from build123d import *

# Parameters (mm, degrees)
SKETCH1_R           = 213.710950615
BOSS_EXTRUDE1_DEPTH = 12
CUT_EXTRUDE1_START  = -6.405003169
CUT_EXTRUDE1_DEPTH  = 6.405003169
CIRPATTERN1_COUNT   = 5


with BuildPart() as part:
    # Sketch1 → Boss-Extrude1 (new body)
    with BuildSketch(Plane.XY):
        Circle(SKETCH1_R)
    extrude(amount=BOSS_EXTRUDE1_DEPTH)

    # Sketch2 → Cut-Extrude1 (cut)
    with BuildSketch(Plane.XY.offset(12).offset(CUT_EXTRUDE1_START)):
        with BuildLine():
            Line((-47.040542179, 100.736288781), (47.040542179, 100.736288781))
            Line((47.040542179, 100.736288781), (107.884686522, 184.48106902))
            ThreePointArc((107.884686522, 184.48106902), (0, 213.710950615), (-107.884686522, 184.48106902))
            Line((-107.884686522, 184.48106902), (-47.040542179, 100.736288781))
        make_face()
    cut_extrude1 = extrude(amount=CUT_EXTRUDE1_DEPTH, mode=Mode.SUBTRACT)

    # CirPattern1: Cut-Extrude1 ×5 about axis
    cirpattern1_axis = Axis((0, 0, 0), (0, 0, 1))
    for i in range(1, CIRPATTERN1_COUNT):
        add(cut_extrude1.rotate(cirpattern1_axis, i * 360 / CIRPATTERN1_COUNT), mode=Mode.SUBTRACT)


solid = part.part
CAD build for the part. Positions are in the model's coordinates, mm. A direction names the side the tool comes from. Round coordinates to 2 decimals unless told otherwise and drop trailing zeros. Loops run counter-clockwise (first coordinate to the right, second up) from the corner with the lowest first, then second, coordinate; pieces in that order, holes last.
(1) Cut at B-B (x = 0). Give the cut face in (y, z) (3 decimals), plus the area to 3 significant figures.
(2) Which spindle directions (+Z, -Z, +X, -X, +Y, -Y) get a long thin tool onto all of the face, cutting with end or side? Do faces 1 (the flat face through (77.037, 142.022, 8.753)), 2 (the flat face through (-151, 47, 5.595)), 3 (the flat face through (158.88, -29.38, 8.75)), 4 (the flat face through (-92, -129, 5.595)). Say none if no direction does.
(3) Cut at A-A (z = 8.5). Give the cut face in (x, y).
(4) Cut at C-C (y = -40.5). Give the cut face in (x, z) (3 decimals), plus the area to 3 significant figures.
(5) Two-plate mould, pull along X, no slides. Class faces 5 (the flat face through (-3, 3, 0)), 6 (the flat face through (-96.01, 30.5, 8.75)), 7 (the flat face through (-2, 158, 5.595)): +X half, -X half, draft (parallel to the pull), parting line (faces both ways), or undercut.
(6) Wall check: line 1 along Z through (x, y) = (-85, -68.5) (3 decimals); line 2 along X through (y, z) = (-168, 8); line 3 along Y through (x, z) = (-1, 11.25). Give the ranges that are in metal, low to high.
(7) Cut at D-D (x = 153.5). Give the cut face in (y, z) (3 decimals).
(8) Drop flat-ended pins along their axis: pin 1 (1.9 mm diameter, centred on y = -140, z = 8, fed in from +X); pin 2 (1 mm diameter, centred on x = -120.5, y = 53, fed in from +Z) (3 decimals); pin 3 (7 mm diameter, centred on y = -175, z = 8.5, fed in from -X); pin 4 (1.5 mm diameter, centred on x = 35, y = 155, fed in from -Z). Give the stop position or say it passes through.
Findings below:
1. outline: (-213.711, 0) - (213.711, 0) - (213.711, 5.595) - (100.736, 5.595) - (100.736, 12) - (-213.711, 12) - close
1. area: 4,410 mm2
2. face 1: +Z, +Y
2. face 2: +Z, -X
2. face 3: +Z, +X
2. face 4: +Z, -Y
3. outline: (-208.79, -45.6) arc R213.71 ccw to (-195.72, -85.84) - (-97.27, -53.85) - (-21.15, -109.15) - (-21.15, -212.66) arc R213.71 ccw to (21.15, -212.66) - (21.15, -109.15) - (97.27, -53.85) - (195.72, -85.84) arc R213.71 ccw to (208.79, -45.6) - (110.34, -13.61) - (81.27, 75.87) - (142.11, 159.61) arc R213.71 ccw to (107.88, 184.48) - (47.04, 100.74) - (-47.04, 100.74) - (-107.88, 184.48) arc R213.71 ccw to (-142.11, 159.61) - (-81.27, 75.87) - (-110.34, -13.61) - close
4. outline: (-209.838, 0) - (209.838, 0) - (209.838, 5.595) - (193.104, 5.595) - (193.104, 12) - (-193.104, 12) - (-193.104, 5.595) - (-209.838, 5.595) - close
4. area: 4,820 mm2
5. face 5: draft
5. face 6: -X half
5. face 7: undercut
6. line 1: z = 0 to 5.595
6. line 2: x = -21.15 to 21.15
6. line 3: y = -213.71 to 100.74
7. outline: (-148.695, 0) - (148.695, 0) - (148.695, 5.595) - (-27.632, 5.595) - (-27.632, 12) - (-72.119, 12) - (-72.119, 5.595) - (-148.695, 5.595) - close
8. pin 1: stops at x = 21.15
8. pin 2: stops at z = 5.595
8. pin 3: stops at x = -125.41
8. pin 4: stops at z = 0
